from build123d import *

# Parameters (mm, degrees)
SKETCH1_W                       = 49
SKETCH1_H                       = 35
BOSS_EXTRUDE1_DEPTH             = 20
F_3_0MM_DOWEL_HOLE1_D           = 3
F_3_0MM_DOWEL_HOLE1_DEPTH       = 11.098709071
F_3_0MM_DOWEL_HOLE1_CSINK_D     = 3.05
F_3_0MM_DOWEL_HOLE1_CSINK_ANGLE = 90
F_3_0MM_DOWEL_HOLE1_TIP         = 0.901290929
F_3_0MM_DOWEL_HOLE2_D           = 3
F_3_0MM_DOWEL_HOLE2_DEPTH       = 12
F_3_0MM_DOWEL_HOLE2_CSINK_D     = 3.05
F_3_0MM_DOWEL_HOLE2_CSINK_ANGLE = 90
F_3_0MM_DOWEL_HOLE2_TIP         = 0.901290929
F_3_0MM_DOWEL_HOLE3_D           = 3
F_3_0MM_DOWEL_HOLE3_CSINK_D     = 3.05
F_3_0MM_DOWEL_HOLE3_CSINK_ANGLE = 90
SKETCH14_W                      = 8
SKETCH14_H                      = 35
SKETCH14_W_2                    = 20
SKETCH14_H_2                    = 16
SKETCH14_H_3                    = 9
CUT_EXTRUDE3_DEPTH              = 28
SKETCH15_R                      = 5.5
CUT_EXTRUDE4_DEPTH              = 30
FILLET1_R                       = 5


with BuildPart() as part:
    # Sketch1 → Boss-Extrude1 (new body)
    with BuildSketch(Plane(origin=(0, 0, 0), x_dir=(1, 0, 0), z_dir=(0, 1, 0))):
        with Locations((13.974428044, 4.809594096)):
            Rectangle(SKETCH1_W, SKETCH1_H)
    extrude(amount=BOSS_EXTRUDE1_DEPTH)

    # Ø3.0mm Dowel Hole1
    with Locations(Plane(origin=(0, 0, -22.309594096), x_dir=(-1, 0, 0), z_dir=(0, 0, -1))):
        with Locations((-7.474428044, 4)):
            CounterSinkHole(F_3_0MM_DOWEL_HOLE1_D / 2, F_3_0MM_DOWEL_HOLE1_CSINK_D / 2, depth=F_3_0MM_DOWEL_HOLE1_DEPTH, counter_sink_angle=F_3_0MM_DOWEL_HOLE1_CSINK_ANGLE)
            with Locations((0, 0, -(F_3_0MM_DOWEL_HOLE1_DEPTH + F_3_0MM_DOWEL_HOLE1_TIP / 2))):  # 118° drill point
                Cone(0, F_3_0MM_DOWEL_HOLE1_D / 2, F_3_0MM_DOWEL_HOLE1_TIP, mode=Mode.SUBTRACT)

    # Ø3.0mm Dowel Hole2
    with Locations(Plane(origin=(38.474428044, 0, 0), x_dir=(0, 0, -1), z_dir=(1, 0, 0))):
        with Locations((0.809594096, 8)):
            CounterSinkHole(F_3_0MM_DOWEL_HOLE2_D / 2, F_3_0MM_DOWEL_HOLE2_CSINK_D / 2, depth=F_3_0MM_DOWEL_HOLE2_DEPTH, counter_sink_angle=F_3_0MM_DOWEL_HOLE2_CSINK_ANGLE)
            with Locations((0, 0, -(F_3_0MM_DOWEL_HOLE2_DEPTH + F_3_0MM_DOWEL_HOLE2_TIP / 2))):  # 118° drill point
                Cone(0, F_3_0MM_DOWEL_HOLE2_D / 2, F_3_0MM_DOWEL_HOLE2_TIP, mode=Mode.SUBTRACT)

    # Ø3.0mm Dowel Hole3 (through all)
    with Locations(Plane(origin=(0, 0, 0), x_dir=(-1, 0, 0), z_dir=(0, -1, 0))):
        with Locations((-7.474428044, 6.309594096)):
            CounterSinkHole(F_3_0MM_DOWEL_HOLE3_D / 2, F_3_0MM_DOWEL_HOLE3_CSINK_D / 2, counter_sink_angle=F_3_0MM_DOWEL_HOLE3_CSINK_ANGLE)

    # Sketch14 → Cut-Extrude3 (cut)
    with BuildSketch(Plane(origin=(0, 20, 0), x_dir=(1, 0, 0), z_dir=(0, 1, 0))):
        with Locations((-6.525571956, 4.809594096)):
            Rectangle(SKETCH14_W, SKETCH14_H)
        with Locations((28.474428044, 14.309594096)):
            Rectangle(SKETCH14_W_2, SKETCH14_H_2)
        with Locations((28.474428044, -8.190405904)):
            Rectangle(SKETCH14_W_2, SKETCH14_H_3)
    extrude(amount=-CUT_EXTRUDE3_DEPTH, mode=Mode.SUBTRACT)

    # Sketch15 → Cut-Extrude4 (cut)
    with BuildSketch(Plane(origin=(0, 20, 0), x_dir=(1, 0, 0), z_dir=(0, 1, 0))):
        with Locations((7.474428044, -2.690405904)):
            Circle(SKETCH15_R)
    extrude(amount=-CUT_EXTRUDE4_DEPTH, mode=Mode.SUBTRACT)

    # Fillet1
    fillet1_edges = [part.edges().sort_by_distance(p)[0] for p in [
        (18.474428044, 10, -6.309594096),
        (18.474428044, 10, 3.690405904),
    ]]
    fillet(fillet1_edges, radius=FILLET1_R)


solid = part.part
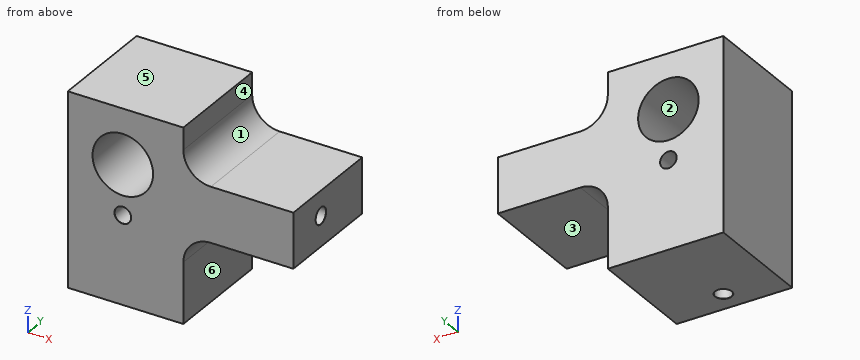
Source: CAD feature listing. Evaluate the final solid. Frame: model axes, mm. Face numbers are marked on the shaded views. A direction names the side the tool comes from. Give positions to 0.01 mm unless a question says otherwise; leave off trailing zeros. Write each loop counter-clockwise with the first axis right and the second up, starting at its lowest first coordinate (ties: lowest second). Pieces come first, ordered by that corner, then holes. Notation, with made-up numbers: M 20,76.5 L 72,76.5 A20 ccw 72,89.5 Z; hole C 89,-39 d6. An arc over 180 degrees is marked long. Return JSON: item names as keys, results as strings. Group by question number.
1) Cut plane C-C, the plane x = 34. Output: boundary loops of the cut face in (y, z), plus the area to 3 significant figures.
2) Pin query (flat end, axial travel): P1, Ø2, axis at y = 14, z = 11, coming from the +X side; P2, Ø1, axis at x = 29, y = 3, coming from the -Z side; P3, Ø7.5, axis at x = 34, y = 10.5, coming from the +Z side. Return the tip coordinate at first contact, or that it passes through.
3) Pull-direction query (X, two-part tool) for the marked faces 1, 2 and 3; classes: pulls with the +X half, pulls with the -X half, needs draft (parallel to the pull), parting line crosses it, or undercut.
4) Material intervals for line 1 along X through (y, z) = (4, -17.25); line 2 along Z through (x, y) = (26, 5); line 3 along X through (y, z) = (8, -1), sorted ascending. Write a range as [from, to].
5) Cut plane D-D, the plane z = 9.5. Output: boundary loops of the cut face in (x, y).
6) Set-up query: the marked faces 4, 5 and 6. Return all of +Z, -Z, +X, -X, +Y, -Y with unobstructed straight access to the full face (end or side cutting, diameter ignored); none if empty.
7) Cut plane A-A, the plane z = -19.5. Output: boundary loops of the cut face in (x, y).
8) Cut plane B-B, the plane y = 17.75. Output: boundary loops of the cut face in (x, z), plus the area to 3 significant figures.
Recorded:
{
 "1": {"outline": "M 0,-6.31 L 20,-6.31 L 20,3.69 L 0,3.69 Z; hole C 8,-0.81 d3", "area": "193 mm²"},
 "2": {"P1": "stops at x = 18.47", "P2": "stops at z = -6.31", "P3": "stops at z = 3.69"},
 "3": {"face 1": "pulls with the +X half", "face 2": "undercut", "face 3": "needs draft"},
 "4": {"line 1": "x = [-2.53, 5.97], [8.97, 18.47]", "line 2": "z = [-6.31, 3.69]", "line 3": "x = [-2.53, 3.4], [11.55, 25.69]"},
 "5": {"outline": "M -2.53,0 L 18.47,0 L 18.47,20 L -2.53,20 Z"},
 "6": {"face 4": "+Z, +X, +Y, -Y", "face 5": "+Z, +X, -X, +Y, -Y", "face 6": "-Z, +X, +Y, -Y"},
 "7": {"outline": "M -2.53,0 L 18.47,0 L 18.47,20 L -2.53,20 Z; hole C 7.47,4 d3"},
 "8": {"outline": "M -2.53,-22.31 L 18.47,-22.31 L 18.47,-11.31 A5 cw 23.47,-6.31 L 38.47,-6.31 L 38.47,3.69 L 23.47,3.69 A5 cw 18.47,8.69 L 18.47,12.69 L -2.53,12.69 Z; hole C 7.47,2.69 d11; hole C 7.47,-6.31 d3", "area": "844 mm²"}
}
